Can you work these out from the model? Positions are in its coordinate system, mm. Face numbers are marked on the shaded views. A direction names the side the tool comes from. Coordinates: 2 decimals unless noted, no trailing zeros. Loops run counter-clockwise (first coordinate to the right, second up) from the corner with the lowest first, then second, coordinate; pieces in that order, holes last. Notation, with made-up numbers: (10, 10) - (69, 10) arc R13 ccw to (69, 32) - close; hole circle Ø3 at (55.5, -30). An arc over 180 degrees is marked (long way). Put each result on its own line as item: value. Start each with the question number.
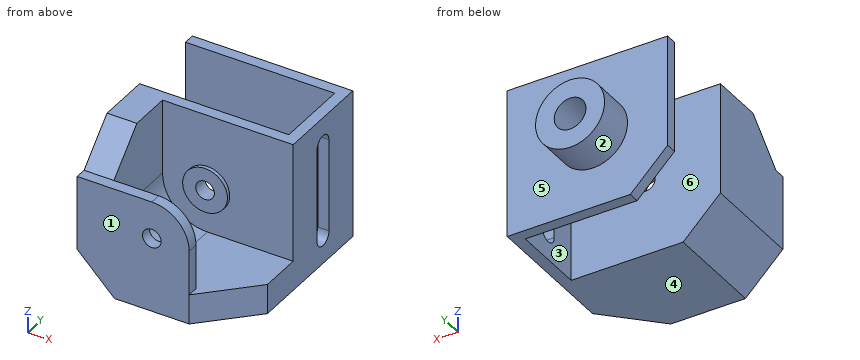
from build123d import *

# Parameters (mm, degrees)
SKETCH1_W           = 40
SKETCH1_H           = 40
SKETCH1_R           = 4.25
BOSS_EXTRUDE1_DEPTH = 3
SKETCH2_R           = 9.25
SKETCH2_R_2         = 4.25
BOSS_EXTRUDE2_DEPTH = 10
SKETCH3_W           = 40
SKETCH3_H           = 23
BOSS_EXTRUDE3_DEPTH = 3
CUT_EXTRUDE1_DEPTH  = 3
SKETCH5_W           = 43
SKETCH5_H           = 40
BOSS_EXTRUDE4_DEPTH = 3
SKETCH6_R           = 2.5
CUT_EXTRUDE2_DEPTH  = 10
SKETCH7_R           = 6
SKETCH7_R_2         = 2.5
BOSS_EXTRUDE5_DEPTH = 1
BOSS_EXTRUDE6_DEPTH = 21.2
CHAMFER2_SIZE       = 10
SKETCH10_R          = 2.5
BOSS_EXTRUDE7_DEPTH = 3
CUT_EXTRUDE3_DEPTH  = 31
BOSS_EXTRUDE8_DEPTH = 8


with BuildPart() as part:
    # Sketch1 → Boss-Extrude1 (new body)
    with BuildSketch(Plane(origin=(0, 0, 0), x_dir=(1, 0, 0), z_dir=(0, 1, 0))):
        Rectangle(SKETCH1_W, SKETCH1_H)
        with Locations(Location((0, 0, 0), (0, 0, 270))):
            Circle(SKETCH1_R, mode=Mode.SUBTRACT)
    extrude(amount=BOSS_EXTRUDE1_DEPTH)

    # Sketch2 → Boss-Extrude2 (add)
    with BuildSketch(Plane(origin=(0, 3, 0), x_dir=(1, 0, 0), z_dir=(0, 1, 0))):
        with Locations(Location((0, 0, 0), (0, 0, 270))):
            Circle(SKETCH2_R)
        with Locations(Location((0, 0, 0), (0, 0, 270))):
            Circle(SKETCH2_R_2, mode=Mode.SUBTRACT)
    extrude(amount=BOSS_EXTRUDE2_DEPTH)

    # Sketch3 → Boss-Extrude3 (add)
    with BuildSketch(Plane(origin=(20, 0, 0), x_dir=(0, 0, -1), z_dir=(1, 0, 0))):
        with Locations((0, -8.5)):
            Rectangle(SKETCH3_W, SKETCH3_H)
    extrude(amount=BOSS_EXTRUDE3_DEPTH)

    # Sketch4 → Cut-Extrude1 (cut)
    with BuildSketch(Plane.ZY.offset(-20)):
        with BuildLine():
            Line((-12.5, -7.4), (12.5, -7.4))
            ThreePointArc((12.5, -7.4), (15.1, -10), (12.5, -12.6))
            Line((12.5, -12.6), (-12.5, -12.6))
            ThreePointArc((-12.5, -12.6), (-15.1, -10), (-12.5, -7.4))
        make_face()
    extrude(amount=-CUT_EXTRUDE1_DEPTH, mode=Mode.SUBTRACT)

    # Sketch5 → Boss-Extrude4 (add)
    with BuildSketch(Plane(origin=(0, -20, 0), x_dir=(-1, 0, 0), z_dir=(0, -1, 0))):
        with Locations((-1.5, 0)):
            Rectangle(SKETCH5_W, SKETCH5_H)
    extrude(amount=BOSS_EXTRUDE4_DEPTH)

    # Sketch6 → Cut-Extrude2 (cut)
    with BuildSketch(Plane(origin=(0, -20, 0), x_dir=(1, 0, 0), z_dir=(0, 1, 0))):
        with Locations(Location((0, 0, 0), (0, 0, 270))):
            Circle(SKETCH6_R)
    extrude(amount=-CUT_EXTRUDE2_DEPTH, mode=Mode.SUBTRACT)

    # Sketch7 → Boss-Extrude5 (add)
    with BuildSketch(Plane(origin=(0, -23, 0), x_dir=(-1, 0, 0), z_dir=(0, -1, 0))):
        with Locations(Location((0, 0, 0), (0, 0, 270))):
            Circle(SKETCH7_R)
        with Locations(Location((0, 0, 0), (0, 0, 270))):
            Circle(SKETCH7_R_2, mode=Mode.SUBTRACT)
    extrude(amount=BOSS_EXTRUDE5_DEPTH)

    # Sketch9 → Boss-Extrude6 (add)
    with BuildSketch(Plane.XZ.offset(23)):
        with BuildLine():
            Line((23, -12), (0, -12))
            ThreePointArc((0, -12), (-8.485281374, -8.485281374), (-12, 0))
            Line((-12, 0), (-12, 20))
            Line((-12, 20), (-20, 20))
            Line((-20, 20), (-20, -10))
            Line((-20, -10), (-10, -20))
            Line((-10, -20), (23, -20))
            Line((23, -20), (23, -12))
        make_face()
    extrude(amount=BOSS_EXTRUDE6_DEPTH)

    # Chamfer2
    chamfer2_edges = [part.edges().sort_by_distance(p)[0] for p in [
        (-16, -44.2, 20),
        (23, -44.2, -16),
    ]]
    chamfer(chamfer2_edges, length=CHAMFER2_SIZE)

    # Sketch10 → Boss-Extrude7 (add)
    with BuildSketch(Plane.XZ.offset(44.2)):
        with BuildLine():
            Line((0, 10), (-12, 10))
            Line((-12, 10), (-20, 10))
            Line((-20, 10), (-20, -10))
            Line((-20, -10), (-10, -20))
            Line((-10, -20), (10, -20))
            Line((10, -20), (10, 0))
            ThreePointArc((10, 0), (7.071067812, 7.071067812), (0, 10))
        make_face()
        with Locations(Location((0, 0, 0), (0, 0, 90))):
            Circle(SKETCH10_R, mode=Mode.SUBTRACT)
    extrude(amount=BOSS_EXTRUDE7_DEPTH)

    # Sketch11 → Cut-Extrude3 (cut)
    with BuildSketch(Plane.XZ.offset(23)):
        Polygon((-10, -20), (-20, -10), (-20, -20), align=None)
    extrude(amount=-CUT_EXTRUDE3_DEPTH, mode=Mode.SUBTRACT)

    # Sketch12 → Boss-Extrude8 (add)
    with BuildSketch(Plane(origin=(0, 0, -20), x_dir=(-1, 0, 0), z_dir=(0, 0, -1))):
        Polygon((-10, -47.2), (-13, -44.2), (-10, -44.2), align=None)
    extrude(amount=-BOSS_EXTRUDE8_DEPTH)


solid = part.part
Q1. I want a section at D-D on y = -38. List the corners of the cut face in (x, z) for me, and give its area (3 significant figures).
Q2. I want a section at A-A on x = 13.5. List the corners of the cut face in (y, z) for me, and give its area (3 significant figures).
Q3. Please list where these lines run through material, in increasing order: line 1 along Y through (x, z) = (-9.5, -2); line 2 along Y through (x, z) = (-1, 5); line 3 along Y through (x, z) = (8, 14.5). Write a range as [from, to].
Q4. I want a section at B-B on y = -10. List the corners of the cut face in (x, z) for me, and give its area (3 significant figures).
Q5. On a 3-axis mill with a long thin cutter (end or side, diameter ignored), from which of +Z, -Z, +X, -X, +Y, -Y can I reach the whole of each face in a straight line? I mean the marked faces 4, 5 and 6. Say none if no direction works.
Q6. I want a section at C-C on z = 8.5. List the corners of the cut face in (x, y) for me, and give its area (3 significant figures).
Q7. Will these pins go through, and if not, where does the flat tip stop? pin 1 (3 mm diameter, centred on x = 15, z = -9, fed in from -Y); pin 2 (3.5 mm diameter, centred on y = -45.5, z = -8, fed in from +X); pin 3 (6 mm diameter, centred on y = -7, z = 12.5, fed in from -X).
Q8. We'd pull the mould along Y, two halves only. Please class the marked faces 1, 2 and 3: released by +Y, released by -Y, zero draft, split by the parting line, or undercut.
Calculated:
1. outline: (-20, -10) - (-10, -20) - (19.2, -20) - (19.2, -12) - (0, -12) arc R12 cw to (-12, 0) - (-12, 16.2) - (-20, 16.2) - close
1. area: 520 mm2
2. outline: (-43.7, -20) - (-20, -20) - (-20, 20) - (-23, 20) - (-23, -12) - (-43.7, -12) - close; (0, -20) - (3, -20) - (3, 20) - (0, 20) - close
2. area: 406 mm2
3. line 1: [-47.2, -44.2], [-23, -20], [0, 3]
3. line 2: [-47.2, -44.2], [-24, -20], [0, 13]
3. line 3: [-23, -20], [0, 3]
4. outline: (20, -20) - (23, -20) - (23, -15.1) - (20, -15.1) - close; (20, 15.1) - (23, 15.1) - (23, 20) - (20, 20) - close
4. area: 29.4 mm2
5. face 4: -Z, +X, -X, +Y, -Y
5. face 5: +Y
5. face 6: +Z, -Z, -X
6. outline: (-20, -47.2) - (5.27, -47.2) - (5.27, -44.2) - (-12, -44.2) - (-12, -23) - (23, -23) - (23, -12.6) - (20, -12.6) - (20, -20) - (-20, -20) - close; (-20, 0) - (20, 0) - (20, -7.4) - (23, -7.4) - (23, 3) - (3.65, 3) - (3.65, 13) - (-3.65, 13) - (-3.65, 3) - (-20, 3) - close
6. area: 621 mm2
7. pin 1: y = -23
7. pin 2: x = 10
7. pin 3: x = 20
8. face 1: released by -Y
8. face 2: zero draft
8. face 3: undercut
